Model file for the job. Use its own axes, mm. A direction names the side the tool comes from. Round coordinates to 2 decimals unless told otherwise and drop trailing zeros. Loops run counter-clockwise (first coordinate to the right, second up) from the corner with the lowest first, then second, coordinate; pieces in that order, holes last. Notation, with made-up numbers: M 60,78 L 70,78 A15 cw 70,90 Z; hole C -28.5,26 d2. An arc over 180 degrees is marked long. Use a Markdown table: item, result. Add a question column.
Item 1: Two-plate mould, pull along Y, no slides. Class faces 4 (the cylindrical face through (-0.78, -12.95, 29.46)), 5 (the flat face through (0, -4.6, 43)), 6 (the flat face through (-15, 0, 0)): +Y half, -Y half, draft (parallel to the pull), parting line (faces both ways), or undercut.
Item 2: Saw through at B-B on z = 2. Write the cut outline in (x, y), then the cut area to 3 significant figures.
Item 3: Pin check, flat tips, straight feed: P1, Ø2.5, axis at x = 15.5, y = 0, coming from the +Z side; P2, Ø2, axis at x = -5.5, y = 13, coming from the +Z side; P3, Ø1, axis at y = 8.5, z = -16, coming from the +X side. Stop position of each tip, or through.
Item 4: Tool access for faces 1 (the flat face through (0, -7, 48.5)), 2 (the cylindrical face through (-9.139, -14.334, -22.185)), 3 (the flat face through (0, 4, 24.5)): list every direction of +Z, -Z, +X, -X, +Y, -Y with a clear straight run to the whole face (end or side of a thin tool).
Item 5: Saw through at C-C on z = 40. Write the cut outline in (x, y), then the cut area to 3 significant figures.
Item 6: Wall check: L1, parallel to X at y = 13.5, z = 7; L2, parallel to Y at x = 7.75, z = 15.25; L3, parallel to Y at x = 0, z = 25.6. Give the ranges that are in metal, low to high. Write a range as from..to.
Item 7: Saw through at D-D on x = -16. Write the cut outline in (y, z).
Item 8: Saw through at A-A on x = 0. Write the cut outline in (y, z), then the cut area to 3 significant figures.
Autodesk Inventor part; units mm, degrees
ref_plane "YZ Plane" through (0, 0, 0) normal (1, 0, 0) x (0, 1, 0)
ref_plane "XZ Plane" through (0, 0, 0) normal (0, 1, 0) x (-1, 0, 0)
ref_plane "XY Plane" through (0, 0, 0) normal (0, 0, 1) x (1, 0, 0)
sketch "Sketch1" plane through (0, 0, 0) normal (0, 0, 1) x (1, 0, 0)
  circle A0 centre (0, 0) radius 18.4
  dimension "d0" = 36.8
extrude "Extrusion1" add sketch "Sketch1" along normal blind 26.5
sketch "Sketch2" plane through (0, 0, 26.5) normal (0, 0, 1) x (1, 0, 0)
  circle A0 centre (0, -7) radius 6
  point P0 (0, 0)
  dimension "d3" = 7
  dimension "d4" = 12
extrude "Extrusion2" add sketch "Sketch2" along normal blind 6
sketch "Sketch3" plane through (0, -7, 32.5) normal (0, 0, 1) x (1, 0, 0)
  circle A0 centre (0, 0) radius 3
  point P0 (0, 7)
  dimension "d7" = 6
extrude "Extrusion3" add sketch "Sketch3" along normal blind 16
sketch "Sketch4" plane through (0, -7, 48.5) normal (0, 0, 1) x (1, 0, 0)
  line L0 (-1.8, 2.4) -> (1.8, 2.4)
  circle A0 centre (0, 0) radius 3
  point P0 (0, 7)
  dimension "d10" = 5.4
extrude "Extrusion4" cut sketch "Sketch4" against normal blind 12 contours A0 L0 picked at (0, 2.6)
sketch "Sketch5" plane through (0, 0, 26.5) normal (0, 0, 1) x (1, 0, 0)
  circle A0 centre (0, 0) radius 18.4
  circle A1 centre (0, 0) radius 12.9
  arc A2 (-1.8, -4.6) -> (1.8, -4.6) centre (0, -7) ccw
  circle A3 centre (0, -7) radius 8.5
  point P0 (-7.8641, -10.2257)
  point P1 (7.8641, -10.2257)
  dimension "d13" = 5.5
  dimension "d14" = 17
extrude "Extrusion5" cut sketch "Sketch5" against normal blind 2 contours A1 A3 picked at (-0.0498, 9.0288)
fillet "Fillet1" radius 0.5 4 edges at (0, 12.9, 24.5) (0, 12.9, 26.5) (0, 1.5, 26.5) (0, 1.5, 24.5)
sketch "Sketch6" plane through (0, 0, 26.5) normal (0, 0, 1) x (1, 0, 0)
  circle A0 centre (-15.5, 0) radius 1.5
  circle A1 centre (-7.75, -13.4234) radius 1.5
  circle A2 centre (7.75, -13.4234) radius 1.5
  circle A3 centre (15.5, 0) radius 1.5
  circle A4 centre (7.75, 13.4234) radius 1.5
  circle A5 centre (-7.75, 13.4234) radius 1.5
  point P0 (0, 0)
  point P1 (0, 0)
  dimension "d18" = 3
  dimension "d21" = 360
  dimension "d23" = 31
extrude "Extrusion6" cut sketch "Sketch6" against normal through all
sketch "Sketch7" plane through (0, 0, 0) normal (0, 0, -1) x (-1, 0, 0)
  circle A0 centre (0, 0) radius 18.4
  circle A1 centre (0, 0) radius 18.4
  circle A2 centre (0, 0) radius 17
  dimension "d26" = 34
extrude "Extrusion7" add sketch "Sketch7" along normal blind 45 contours A2
properties part number "37D mm Metal Gearbox Polulu" material "Stainless Steel"
Entries:
| question | item | result |
|---|---|---|
| 1 | face 4 | parting line |
| 1 | face 5 | +Y half |
| 1 | face 6 | undercut |
| 2 | outline | C 0,0 d36.8; hole C -15.5,0 d3; hole C -7.75,-13.42 d3; hole C -7.75,13.42 d3; hole C 7.75,-13.42 d3; hole C 7.75,13.42 d3; hole C 15.5,0 d3 |
| 2 | area | 1,020 mm2 |
| 3 | P1 | z = 0 |
| 3 | P2 | z = 26.5 |
| 3 | P3 | x = 15 |
| 4 | face 1 | +Z, +X, -X, +Y, -Y |
| 4 | face 2 | -Z |
| 4 | face 3 | +Z |
| 5 | outline | M -1.8,-4.6 A3 ccw long 1.8,-4.6 Z |
| 5 | area | 26.8 mm2 |
| 6 | L1 | -12.5..-9.25, -6.25..6.25, 9.25..12.5 |
| 6 | L2 | -16.69..-14.92, -11.92..11.92, 14.92..16.69 |
| 6 | L3 | -18.4..1.5, 12.9..18.4 |
| 7 | outline | M -9.09,0 L -5.74,0 L -5.74,-45 L 5.74,-45 L 5.74,0 L 9.09,0 L 9.09,26.5 L 1.41,26.5 L 1.41,0 L -1.41,0 L -1.41,26.5 L -9.09,26.5 Z |
| 8 | outline | M -18.4,0 L -17,0 L -17,-45 L 17,-45 L 17,0 L 18.4,0 L 18.4,26.5 L 13.4,26.5 A0.5 ccw 12.9,26 L 12.9,25 A0.5 cw 12.4,24.5 L 2,24.5 A0.5 cw 1.5,25 L 1.5,26 A0.5 ccw 1,26.5 L -1,26.5 L -1,32.5 L -4,32.5 L -4,36.5 L -4.6,36.5 L -4.6,48.5 L -10,48.5 L -10,32.5 L -13,32.5 L -13,26.5 L -18.4,26.5 Z |
| 8 | area | 2,640 mm2 |
